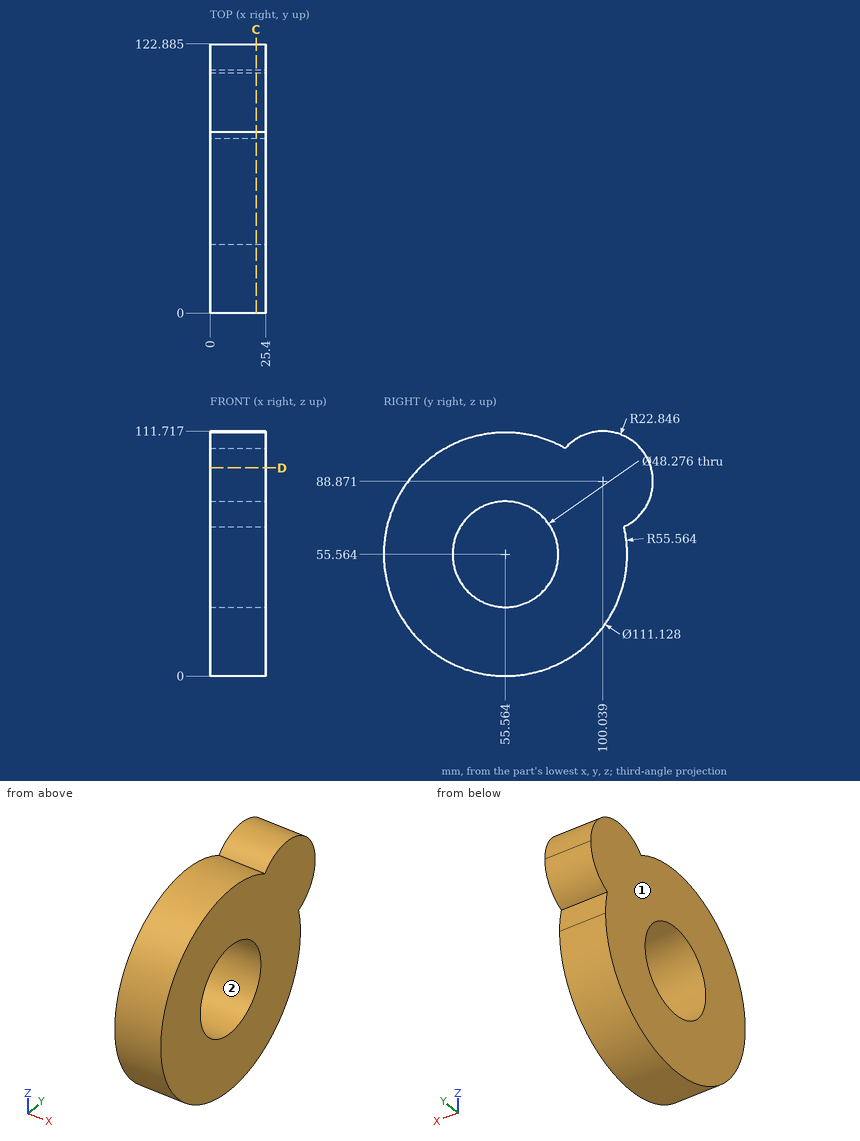
Here's the drawing with two shaded views (mm, measured from the low corner). I have some questions. Coordinates: 2 decimals unless noted, no trailing zeros. Loops run counter-clockwise (first coordinate to the right, second up) from the corner with the lowest first, then second, coordinate; pieces in that order, holes last. Notation, with made-up numbers: (53.25, 87) -> (90.25, 87) arc R29 ccw to (90.25, 108) -> close; hole circle Ø11 at (26, 0.5). An arc over 180 degrees is marked (long way). Put each result on its own line as item: value. Start each with the question number.
Q1. If I drill on line 1 (Y direction, x = 3, z = 71) (1 decimal); line 2 (Y direction, x = 22, z = 61.5); line 3 (Z direction, x = 13.5, y = 61) (1 decimal), over which ranges is the centre line in solid material (lowest first)? Write a range as [from, to].
Q2. I'm going to push flat-ended pins straight in: P1, Ø2, axis at x = 11, y = 28.5, coming from the -Z side; P2, Ø1.5, axis at x = 10, z = 29, coming from the -Y side; P3, Ø6, axis at x = 21.5, z = 35, coming from the +Y side. Where does each tip first touch, or does it pass through?
Q3. I want a section at D-D (z = 95). Write out the boundary of the cut face in (x, y), plus the area to 3 significant figures.
Q4. Thinking about a two-plate mould opening in Y: for the marked faces 1 and 2, which applies, pulls with the +Y half, pulls with the -Y half, needs draft (parallel to the pull), parting line crosses it, or undercut?
Q5. I want a section at C-C (x = 21). Write out the boundary of the cut face in (y, z) (1 decimal).
Taken from the geometry:
1. line 1: y = [2.2, 37], [74.1, 114.3]
1. line 2: y = [0.32, 32.17], [78.96, 110.81]
1. line 3: z = [0.3, 32], [79.1, 110.9]
2. P1: stops at z = 6.49
2. P2: stops at y = 6.36
2. P3: stops at y = 108.28
3. outline: (0, 16.42) -> (25.4, 16.42) -> (25.4, 122.05) -> (0, 122.05) -> close
3. area: 2,680 mm2
4. face 1: needs draft
4. face 2: undercut
5. outline: (82.9, 104) arc R55.6 ccw (long way) to (109.7, 68.2) arc R22.8 ccw (long way) to start; hole circle Ø48.3 at (55.6, 55.6)
